Work out the finished part from the listing and answer in its coordinate system (mm). Face numbers are marked on the shaded views. A direction names the side the tool comes from. Coordinates: 2 decimals unless noted, no trailing zeros. Loops run counter-clockwise (first coordinate to the right, second up) from the corner with the lowest first, then second, coordinate; pieces in that order, holes last. Notation, with made-up numbers: (68, 70) -> (126, 70) arc R24 cw to (126, 100) -> close; hole circle Ø11 at (69.5, 25.5). An arc over 180 degrees is marked (long way). Use a Markdown table: item, result. Add a question column.
```python
from build123d import *

# Parameters (mm, degrees)
SKETCH1_R                    = 2
SKETCH1_R_2                  = 1
SKETCH1_W                    = 22.5
SKETCH1_H                    = 12
BASE_FLANGE1_DEPTH           = 1.5875
EDGE_FLANGE1_STRIP_W         = 7.8232
EDGE_FLANGE1_STRIP_H         = 1.5875
EDGE_FLANGE1_STRIP_CUT_DEPTH = 40
EDGE_FLANGE1_DEPTH           = 40
EDGE_FLANGE1_PROFILE_W       = 60
EDGE_FLANGE1_PROFILE_H       = 15.2634
EDGE_FLANGE1_FLAT_DEPTH      = 1.5875
SKETCH11_R                   = 2
SKETCH11_R_2                 = 1
CUT_EXTRUDE1_DEPTH           = 61.789967563
EDGE_FLANGE2_STRIP_W         = 7.8232
EDGE_FLANGE2_STRIP_H         = 1.5875
EDGE_FLANGE2_STRIP_CUT_DEPTH = 15.2634
EDGE_FLANGE2_DEPTH           = 15.2634
SKETCH15_R                   = 2
CUT_EXTRUDE2_DEPTH           = 73.755464786


# Sheet-metal steps are written as plain solids
with BuildPart() as part:
    # Sketch1 → Base-Flange1 (new body)
    with BuildSketch(Plane(origin=(0, 0, 0), x_dir=(1, 0, 0), z_dir=(0, 1, 0))):
        Polygon((0, 0), (17.5, 0), (17.5, -23.5), (-22.5, -23.5), (-22.5, 10.128421097), (-8, 18.5), (0, 18.5), align=None)
        with Locations(Location((-8, 10.5, 0), (0, 0, 270))):
            Circle(SKETCH1_R, mode=Mode.SUBTRACT)
        with Locations(Location((11.75, -11.75, 0), (0, 0, 270))):
            Circle(SKETCH1_R_2, mode=Mode.SUBTRACT)
        with Locations(Location((-15.25, -11.75, 0), (0, 0, 270))):
            Circle(SKETCH1_R_2, mode=Mode.SUBTRACT)
        with Locations((-1.75, -11.75)):
            Rectangle(SKETCH1_W, SKETCH1_H, mode=Mode.SUBTRACT)
    extrude(amount=-BASE_FLANGE1_DEPTH)

    # Edge-Flange1 strip (across the edge) → Edge-Flange1 strip cut (cut)
    with BuildSketch(Plane(origin=(-22.5, 0, 23.5), x_dir=(0, 0, -1), z_dir=(1, 0, 0))):
        with Locations((-1.5875, -0.79375)):
            Rectangle(EDGE_FLANGE1_STRIP_W, EDGE_FLANGE1_STRIP_H)
    extrude(amount=EDGE_FLANGE1_STRIP_CUT_DEPTH, mode=Mode.SUBTRACT)

    # Edge-Flange1 bend section (across the edge) → Edge-Flange1 (add)
    with BuildSketch(Plane(origin=(-22.5, 0, 23.5), x_dir=(0, 0, -1), z_dir=(1, 0, 0))):
        with BuildLine():
            Line((0, 0.7366), (1.5875, 0.7366))
            ThreePointArc((1.5875, 0.7366), (1.803245145, 0.215745145), (2.3241, 0))
            Line((2.3241, 0), (2.3241, -1.5875))
            ThreePointArc((2.3241, -1.5875), (0.68071313, -0.90678687), (0, 0.7366))
        make_face()
    extrude(amount=EDGE_FLANGE1_DEPTH)

    # Edge-Flange1 profile (on flange) → Edge-Flange1 flat (add)
    with BuildSketch(Plane.XY.offset(23.5)):
        with Locations((-12.5, 8.3683)):
            Rectangle(EDGE_FLANGE1_PROFILE_W, EDGE_FLANGE1_PROFILE_H)
    extrude(amount=-EDGE_FLANGE1_FLAT_DEPTH)

    # Sketch11 → Cut-Extrude1 (cut, through all)
    with BuildSketch(Plane(origin=(0, 0, 21.9125), x_dir=(-1, 0, 0), z_dir=(0, 0, -1))):
        with Locations((12.5, 8.3683)):
            Circle(SKETCH11_R)
        with Locations((26.5, 8.3683)):
            Circle(SKETCH11_R_2)
    extrude(amount=-CUT_EXTRUDE1_DEPTH, mode=Mode.SUBTRACT)

    # Edge-Flange2 strip (across the edge) → Edge-Flange2 strip cut (cut)
    with BuildSketch(Plane(origin=(-42.5, 16, 23.5), x_dir=(1, 0, 0), z_dir=(0, -1, 0))):
        with Locations((-1.5875, -0.79375)):
            Rectangle(EDGE_FLANGE2_STRIP_W, EDGE_FLANGE2_STRIP_H)
    edge_flange2_strip_cut = extrude(amount=EDGE_FLANGE2_STRIP_CUT_DEPTH, mode=Mode.SUBTRACT)

    # Edge-Flange2 section (across the edge) → Edge-Flange2 (add)
    with BuildSketch(Plane(origin=(-42.5, 16, 23.5), x_dir=(1, 0, 0), z_dir=(0, -1, 0))):
        with BuildLine():
            Line((0, 0.7366), (0, 14.4125))
            Line((0, 14.4125), (1.5875, 14.4125))
            Line((1.5875, 14.4125), (1.5875, 0.7366))
            ThreePointArc((1.5875, 0.7366), (1.803245145, 0.215745145), (2.3241, 0))
            Line((2.3241, 0), (2.3241, -1.5875))
            ThreePointArc((2.3241, -1.5875), (0.68071313, -0.90678687), (0, 0.7366))
        make_face()
    edge_flange2 = extrude(amount=EDGE_FLANGE2_DEPTH)

    # Sketch15 → Cut-Extrude2 (cut, through all)
    with BuildSketch(Plane.ZY.offset(42.5)):
        with Locations((31.07455, 8)):
            Circle(SKETCH15_R)
    cut_extrude2 = extrude(amount=-CUT_EXTRUDE2_DEPTH, mode=Mode.SUBTRACT)

    # Mirror1: Edge-Flange2 strip cut, Edge-Flange2, Cut-Extrude2 across plane
    add(edge_flange2_strip_cut.mirror(Plane.ZY.offset(12.5)), mode=Mode.SUBTRACT)
    add(edge_flange2.mirror(Plane.ZY.offset(12.5)))
    add(cut_extrude2.mirror(Plane.ZY.offset(12.5)), mode=Mode.SUBTRACT)


solid = part.part
```
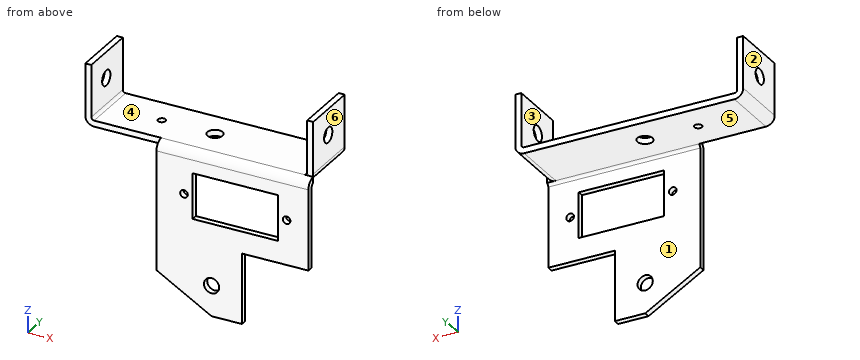
Item 1: Given pin 1 (6 mm diameter, centred on x = -35.5, y = 14, fed in from -Z); pin 2 (7.5 mm diameter, centred on x = -15, y = 8.5, fed in from +Z); pin 3 (0.7 mm diameter, centred on y = -0.5, z = 9, fed in from -X); pin 4 (1.3 mm diameter, centred on x = 0.5, y = -1, fed in from -Z), each flat-ended and moving along its own axis, determine where each tip first touches the part or whether it passes through.
Item 2: For the marked faces 4, 5 and 6, determine the directions among +Z, -Z, +X, -X, +Y, -Y from which every point of the face is accessible in a straight line to the end or side of a thin tool.
Item 3: Section C-C (y = 4.75) is taken. Determine the outline of the cut face in (x, z), then the cut area to 3 significant figures.
Item 4: For a pull along X with two mould halves and no side action, classify the marked faces 1, 2 and 3 as +X half, -X half, draft (parallel to the pull), parting line (faces both ways), or undercut.
Item 5: Section B-B (z = 26.5) is taken. Determine the outline of the cut face in (x, y).
Item 6: Section A-A (x = 4.5) is taken. Determine the outline of the cut face in (y, z).
Item 7: Section D-D (x = 11.75) is taken. Determine the outline of the cut face in (y, z), then the cut area to 3 significant figures.
Item 8: Find the intervals of material crossed by probe 1 along X at (y, z) = (7.75, 29); probe 2 along X at (y, z) = (-0.9, 11.75); probe 3 along Z at (x, y) = (-21, 15), in increasing order.
Output:
| question | item | result |
|---|---|---|
| 1 | pin 1 | stops at z = 21.91 |
| 1 | pin 2 | stops at z = 23.5 |
| 1 | pin 3 | stops at x = -22.5 |
| 1 | pin 4 | stops at z = -18.5 |
| 2 | face 4 | +Z, +Y, -Y |
| 2 | face 5 | -Z, +X, -X, +Y |
| 2 | face 6 | +Z, -Z, +X, +Y, -Y |
| 3 | outline | (-42.5, 24.24) arc R2.32 ccw to (-40.18, 21.91) -> (15.18, 21.91) arc R2.32 ccw to (17.5, 24.24) -> (17.5, 37.91) -> (15.91, 37.91) -> (15.91, 24.24) arc R0.74 cw to (15.18, 23.5) -> (-40.18, 23.5) arc R0.74 cw to (-40.91, 24.24) -> (-40.91, 37.91) -> (-42.5, 37.91) -> close |
| 3 | area | 139 mm2 |
| 4 | face 1 | draft |
| 4 | face 2 | -X half |
| 4 | face 3 | undercut |
| 5 | outline | (-42.5, 0.74) -> (-40.91, 0.74) -> (-40.91, 16) -> (-42.5, 16) -> close; (15.91, 0.74) -> (17.5, 0.74) -> (17.5, 16) -> (15.91, 16) -> close |
| 6 | outline | (-1.59, 0) -> (0, 0) -> (0, 5.75) -> (-1.59, 5.75) -> close; (-1.59, 17.75) -> (0, 17.75) -> (0, 21.18) arc R0.74 cw to (0.74, 21.91) -> (16, 21.91) -> (16, 23.5) -> (0.74, 23.5) arc R2.32 ccw to (-1.59, 21.18) -> close |
| 7 | outline | (-1.59, 0) -> (0, 0) -> (0, 10.75) -> (-1.59, 10.75) -> close; (-1.59, 12.75) -> (0, 12.75) -> (0, 21.18) arc R0.74 cw to (0.74, 21.91) -> (16, 21.91) -> (16, 23.5) -> (0.74, 23.5) arc R2.32 ccw to (-1.59, 21.18) -> close |
| 7 | area | 58.5 mm2 |
| 8 | probe 1 | x = -42.5 to -40.91, 15.91 to 17.5 |
| 8 | probe 2 | x = -22.5 to -16.25, -14.25 to -13, 9.5 to 10.75, 12.75 to 17.5 |
| 8 | probe 3 | z = 21.91 to 23.5 |
